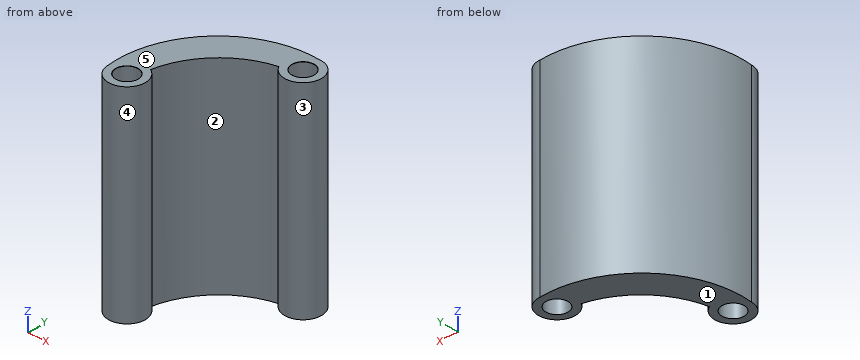
```python
from build123d import *

# Parameters (mm, degrees)
BOSS_EXTRUDE1_DEPTH             = 27.94
F_3_0MM_DOWEL_HOLE1_D           = 3
F_3_0MM_DOWEL_HOLE1_CSINK_D     = 3.05
F_3_0MM_DOWEL_HOLE1_CSINK_ANGLE = 100


with BuildPart() as part:
    # Sketch1 → Boss-Extrude1 (new body)
    with BuildSketch(Plane(origin=(0, 0, 0), x_dir=(0, 1, 0), z_dir=(0, 0, 1))):
        with BuildLine():
            ThreePointArc((0, 15), (-2.153485547, 11.23015749), (2.187669993, 11.29))
            ThreePointArc((2.187669993, 11.29), (8.131727984, 8.131727984), (11.29, 2.187669993))
            ThreePointArc((11.29, 2.187669993), (11.23015749, -2.153485547), (15, 0))
            ThreePointArc((15, 0), (11.072722586, 11.072722586), (0, 15))
        make_face()
    extrude(amount=BOSS_EXTRUDE1_DEPTH)

    # Ø3.0mm Dowel Hole1 (through all)
    with Locations(Plane.XY.offset(27.94)):
        with Locations((0, 12.5), (0, -12.5), (-12.5, 0)):
            CounterSinkHole(F_3_0MM_DOWEL_HOLE1_D / 2, F_3_0MM_DOWEL_HOLE1_CSINK_D / 2, counter_sink_angle=F_3_0MM_DOWEL_HOLE1_CSINK_ANGLE)


solid = part.part
```
Source: CAD feature listing. Evaluate the final solid. Frame: model axes, mm. Face numbers are marked on the shaded views. A direction names the side the tool comes from. Coordinates: 2 decimals unless noted, no trailing zeros. Loops run counter-clockwise (first coordinate to the right, second up) from the corner with the lowest first, then second, coordinate; pieces in that order, holes last. Notation, with made-up numbers: (-28.5, 61.25) -> (23.5, 61.25) arc R25 ccw to (23.5, 79.25) -> close; hole circle Ø8 at (0.25, -2.75). An arc over 180 degrees is marked (long way). One line per item, written item: value. Start each with the question number.
Q1. Section query C-C, the plane y = 12.5. Return the cut outline in (x, z) (3 decimals), and give its area (3 significant figures).
Q2. Section query B-B, the plane x = -12.5. Return the cut outline in (y, z) (3 decimals).
Q3. Section query D-D, the plane y = 8.25. Return the cut outline in (x, z).
Q4. Line query: line 1 along Y through (x, z) = (-13, 17); line 2 along Y through (x, z) = (-10.5, 7.5); line 3 along X through (y, z) = (12.5, 18). Output: solid intervals per line, ascending.
Q5. Contact query for flat-ended pins moving along their axis: P1, Ø1.5, axis at x = 0, z = 3, coming from the -Y side; P2, Ø6, axis at x = -6, z = 5.5, coming from the +Y side; P3, Ø1.5, axis at x = -12, z = 18.5, coming from the +Y side. Output: stop coordinate, or through.
Q6. Set-up query: the marked faces 1 and 2. Return all of +Z, -Z, +X, -X, +Y, -Y with unobstructed straight access to the full face (end or side cutting, diameter ignored); none if empty.
Q7. Section query A-A, the plane z = 25.75. Return the cut outline in (x, y).
Q8. Mould query, pull axis X, two halves, no side actions, for the marked faces 3, 4 and 5. Classes: pulls with the +X half, pulls with the -X half, needs draft (parallel to the pull), parting line crosses it, or undercut.
Results:
1. outline: (-9.394, 0) -> (-1.5, 0) -> (-1.5, 27.919) -> (-1.525, 27.94) -> (-9.394, 27.94) -> close; (1.5, 0) -> (2.5, 0) -> (2.5, 27.94) -> (1.525, 27.94) -> (1.5, 27.919) -> close
1. area: 249 mm^2
2. outline: (-2.5, 0) -> (-1.5, 0) -> (-1.5, 27.919) -> (-1.525, 27.94) -> (-2.5, 27.94) -> close; (1.5, 0) -> (9.394, 0) -> (9.394, 27.94) -> (1.525, 27.94) -> (1.5, 27.919) -> close
3. outline: (-13.24, 0) -> (-8.01, 0) -> (-8.01, 27.94) -> (-13.24, 27.94) -> close
4. line 1: -2.45 to -1.41, 1.41 to 8.65
4. line 2: -1.5 to 1.5, 4.69 to 11.61
4. line 3: -9.39 to -1.5, 1.5 to 2.5
5. P1: y = 10
5. P2: y = 14.98
5. P3: y = 10.89
6. face 1: -Z, +X, -X, +Y, -Y
6. face 2: +Z, -Z
7. outline: (-15, 0) arc R2.5 ccw (long way) to (-11.29, 2.19) arc R11.5 cw to (-2.19, 11.29) arc R2.5 ccw (long way) to (0, 15) arc R13.66 ccw to start; hole circle Ø3 at (-12.5, 0); hole circle Ø3 at (0, 12.5)
8. face 3: undercut
8. face 4: parting line crosses it
8. face 5: needs draft
